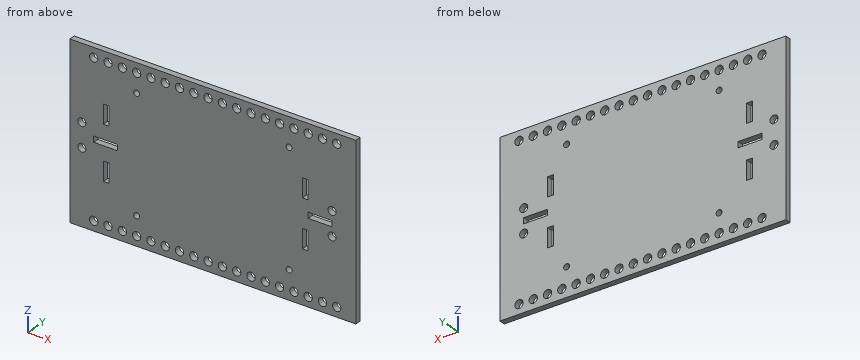
```python
from build123d import *

# Parameters (mm, degrees)
SKETCH1_W           = 152.4
SKETCH1_H           = 91.44
SKETCH1_R           = 2.2225
SKETCH1_R_2         = 2.15265
SKETCH1_R_3         = 1.5875
SKETCH1_W_2         = 12.7
SKETCH1_H_2         = 3.0734
SKETCH1_H_3         = 3.1242
BOSS_EXTRUDE1_DEPTH = 3.175
CUT_EXTRUDE2_REACH  = 90.92
SKETCH2_W           = 3.1242
SKETCH2_H           = 10.1092


with BuildPart() as part:
    # Sketch1 → Boss-Extrude1 (new body)
    with BuildSketch(Plane(origin=(0, 0, 0), x_dir=(1, 0, 0), z_dir=(0, 1, 0))):
        Rectangle(SKETCH1_W, SKETCH1_H)
        with Locations(Location((-63.5, 40.64, 0), (0, 0, 270))):
            Circle(SKETCH1_R, mode=Mode.SUBTRACT)
        with Locations(Location((-63.5, -40.64, 0), (0, 0, 270))):
            Circle(SKETCH1_R, mode=Mode.SUBTRACT)
        with Locations(Location((-69.85, -6.35, 0), (0, 0, 270))):
            Circle(SKETCH1_R_2, mode=Mode.SUBTRACT)
        with Locations(Location((-69.85, 6.35, 0), (0, 0, 270))):
            Circle(SKETCH1_R_2, mode=Mode.SUBTRACT)
        with Locations(Location((63.5, 6.35, 0), (0, 0, 270))):
            Circle(SKETCH1_R_2, mode=Mode.SUBTRACT)
        with Locations(Location((63.5, -6.35, 0), (0, 0, 270))):
            Circle(SKETCH1_R_2, mode=Mode.SUBTRACT)
        with Locations(Location((-55.88, -40.64, 0), (0, 0, 270))):
            Circle(SKETCH1_R, mode=Mode.SUBTRACT)
        with Locations(Location((-55.88, 40.64, 0), (0, 0, 270))):
            Circle(SKETCH1_R, mode=Mode.SUBTRACT)
        with Locations(Location((-48.26, -40.64, 0), (0, 0, 270))):
            Circle(SKETCH1_R, mode=Mode.SUBTRACT)
        with Locations(Location((-48.26, 40.64, 0), (0, 0, 270))):
            Circle(SKETCH1_R, mode=Mode.SUBTRACT)
        with Locations(Location((-40.64, -40.64, 0), (0, 0, 270))):
            Circle(SKETCH1_R, mode=Mode.SUBTRACT)
        with Locations(Location((-40.64, 40.64, 0), (0, 0, 270))):
            Circle(SKETCH1_R, mode=Mode.SUBTRACT)
        with Locations(Location((-33.02, -40.64, 0), (0, 0, 270))):
            Circle(SKETCH1_R, mode=Mode.SUBTRACT)
        with Locations(Location((-33.02, 40.64, 0), (0, 0, 270))):
            Circle(SKETCH1_R, mode=Mode.SUBTRACT)
        with Locations(Location((-25.4, -40.64, 0), (0, 0, 270))):
            Circle(SKETCH1_R, mode=Mode.SUBTRACT)
        with Locations(Location((-25.4, 40.64, 0), (0, 0, 270))):
            Circle(SKETCH1_R, mode=Mode.SUBTRACT)
        with Locations(Location((-17.78, -40.64, 0), (0, 0, 270))):
            Circle(SKETCH1_R, mode=Mode.SUBTRACT)
        with Locations(Location((-17.78, 40.64, 0), (0, 0, 270))):
            Circle(SKETCH1_R, mode=Mode.SUBTRACT)
        with Locations(Location((-10.16, -40.64, 0), (0, 0, 270))):
            Circle(SKETCH1_R, mode=Mode.SUBTRACT)
        with Locations(Location((-10.16, 40.64, 0), (0, 0, 270))):
            Circle(SKETCH1_R, mode=Mode.SUBTRACT)
        with Locations(Location((-2.54, -40.64, 0), (0, 0, 270))):
            Circle(SKETCH1_R, mode=Mode.SUBTRACT)
        with Locations(Location((-2.54, 40.64, 0), (0, 0, 270))):
            Circle(SKETCH1_R, mode=Mode.SUBTRACT)
        with Locations(Location((5.08, -40.64, 0), (0, 0, 270))):
            Circle(SKETCH1_R, mode=Mode.SUBTRACT)
        with Locations(Location((5.08, 40.64, 0), (0, 0, 270))):
            Circle(SKETCH1_R, mode=Mode.SUBTRACT)
        with Locations(Location((12.7, -40.64, 0), (0, 0, 270))):
            Circle(SKETCH1_R, mode=Mode.SUBTRACT)
        with Locations(Location((12.7, 40.64, 0), (0, 0, 270))):
            Circle(SKETCH1_R, mode=Mode.SUBTRACT)
        with Locations(Location((20.32, -40.64, 0), (0, 0, 270))):
            Circle(SKETCH1_R, mode=Mode.SUBTRACT)
        with Locations(Location((20.32, 40.64, 0), (0, 0, 270))):
            Circle(SKETCH1_R, mode=Mode.SUBTRACT)
        with Locations(Location((27.94, -40.64, 0), (0, 0, 270))):
            Circle(SKETCH1_R, mode=Mode.SUBTRACT)
        with Locations(Location((27.94, 40.64, 0), (0, 0, 270))):
            Circle(SKETCH1_R, mode=Mode.SUBTRACT)
        with Locations(Location((35.56, -40.64, 0), (0, 0, 270))):
            Circle(SKETCH1_R, mode=Mode.SUBTRACT)
        with Locations(Location((35.56, 40.64, 0), (0, 0, 270))):
            Circle(SKETCH1_R, mode=Mode.SUBTRACT)
        with Locations(Location((43.18, -40.64, 0), (0, 0, 270))):
            Circle(SKETCH1_R, mode=Mode.SUBTRACT)
        with Locations(Location((43.18, 40.64, 0), (0, 0, 270))):
            Circle(SKETCH1_R, mode=Mode.SUBTRACT)
        with Locations(Location((50.8, -40.64, 0), (0, 0, 270))):
            Circle(SKETCH1_R, mode=Mode.SUBTRACT)
        with Locations(Location((50.8, 40.64, 0), (0, 0, 270))):
            Circle(SKETCH1_R, mode=Mode.SUBTRACT)
        with Locations(Location((58.42, -40.64, 0), (0, 0, 270))):
            Circle(SKETCH1_R, mode=Mode.SUBTRACT)
        with Locations(Location((58.42, 40.64, 0), (0, 0, 270))):
            Circle(SKETCH1_R, mode=Mode.SUBTRACT)
        with Locations(Location((66.04, -40.64, 0), (0, 0, 270))):
            Circle(SKETCH1_R, mode=Mode.SUBTRACT)
        with Locations(Location((66.04, 40.64, 0), (0, 0, 270))):
            Circle(SKETCH1_R, mode=Mode.SUBTRACT)
        with Locations(Location((-40.64, 30.48, 0), (0, 0, 270))):
            Circle(SKETCH1_R_3, mode=Mode.SUBTRACT)
        with Locations(Location((-40.64, -30.48, 0), (0, 0, 270))):
            Circle(SKETCH1_R_3, mode=Mode.SUBTRACT)
        with Locations(Location((40.64, -30.48, 0), (0, 0, 270))):
            Circle(SKETCH1_R_3, mode=Mode.SUBTRACT)
        with Locations(Location((40.64, 30.48, 0), (0, 0, 270))):
            Circle(SKETCH1_R_3, mode=Mode.SUBTRACT)
        with Locations((57.15, 0)):
            Rectangle(SKETCH1_W_2, SKETCH1_H_2, mode=Mode.SUBTRACT)
        with Locations((-57.15, -0.0254)):
            Rectangle(SKETCH1_W_2, SKETCH1_H_3, mode=Mode.SUBTRACT)
    extrude(amount=BOSS_EXTRUDE1_DEPTH)

    # Sketch2 → Cut-Extrude2 (cut, up to next)
    with BuildSketch(Plane(origin=(0, 3.175, 0), x_dir=(1, 0, 0), z_dir=(0, 1, 0)), mode=Mode.PRIVATE) as cut_extrude2_sk1:
        with Locations((-56.8579, 14.2113)):
            Rectangle(SKETCH2_W, SKETCH2_H)
    cut_extrude2_tool1 = extrude(cut_extrude2_sk1.sketch, amount=-CUT_EXTRUDE2_REACH, mode=Mode.PRIVATE) & part.part
    # Sketch2 → Cut-Extrude2 (cut, up to next)
    with BuildSketch(Plane(origin=(0, 3.175, 0), x_dir=(1, 0, 0), z_dir=(0, 1, 0)), mode=Mode.PRIVATE) as cut_extrude2_sk2:
        with Locations((-56.8579, -14.2113)):
            Rectangle(SKETCH2_W, SKETCH2_H)
    cut_extrude2_tool2 = extrude(cut_extrude2_sk2.sketch, amount=-CUT_EXTRUDE2_REACH, mode=Mode.PRIVATE) & part.part
    # Sketch2 → Cut-Extrude2 (cut, up to next)
    with BuildSketch(Plane(origin=(0, 3.175, 0), x_dir=(1, 0, 0), z_dir=(0, 1, 0)), mode=Mode.PRIVATE) as cut_extrude2_sk3:
        with Locations((49.2379, 12.6746)):
            Rectangle(SKETCH2_W, SKETCH2_H)
    cut_extrude2_tool3 = extrude(cut_extrude2_sk3.sketch, amount=-CUT_EXTRUDE2_REACH, mode=Mode.PRIVATE) & part.part
    # Sketch2 → Cut-Extrude2 (cut, up to next)
    with BuildSketch(Plane(origin=(0, 3.175, 0), x_dir=(1, 0, 0), z_dir=(0, 1, 0)), mode=Mode.PRIVATE) as cut_extrude2_sk4:
        with Locations((49.2379, -12.6746)):
            Rectangle(SKETCH2_W, SKETCH2_H)
    cut_extrude2_tool4 = extrude(cut_extrude2_sk4.sketch, amount=-CUT_EXTRUDE2_REACH, mode=Mode.PRIVATE) & part.part
    add(cut_extrude2_tool1.solids().sort_by_distance((-56.8579, 3.175, -14.2113))[0], mode=Mode.SUBTRACT)
    add(cut_extrude2_tool2.solids().sort_by_distance((-56.8579, 3.175, 14.2113))[0], mode=Mode.SUBTRACT)
    add(cut_extrude2_tool3.solids().sort_by_distance((49.2379, 3.175, -12.6746))[0], mode=Mode.SUBTRACT)
    add(cut_extrude2_tool4.solids().sort_by_distance((49.2379, 3.175, 12.6746))[0], mode=Mode.SUBTRACT)


solid = part.part
```
Geometry check sheet. Reference: the model listing, model coordinates, mm. Round coordinates to 2 decimals unless told otherwise and drop trailing zeros. Order: outer loops, then holes, each group sorted by start corner. A loop starts at its lowest first (then second) coordinate and runs counter-clockwise, first axis right, second up. Notation, with made-up numbers: (65, -9.75) - (115, -9.75) arc R27 ccw to (115, 19.25) - close; hole circle Ø1 at (49, 24.5). An arc over 180 degrees is marked (long way). Use a Markdown table: item, result. Add a question column.
1) Section check A-A (x = 12.7). Record the cut outline in (y, z) (1 decimal).
2) Section check B-B (x = 58.42). Record the cut outline in (y, z) (1 decimal).
3) Section check C-C (z = -14.5). Record the cut outline in (x, y) (3 decimals), then the cut area to 3 significant figures.
4) Section check D-D (y = 1.05). Count the separate pieces of the cut face and the enclosed holes in it, then the cut area to 3 significant figures.
5) Gauge pin test, flat ends, axial feed: P1, Ø8, axis at x = -22.5, z = -4.5, coming from the -Y side; P2, Ø3.5, axis at x = -17.78, z = -40.64, coming from the -Y side. Record the tip position at first contact, or that the pin passes through.
6) Thickness scan on line 1 along Z through (x, y) = (66, 1); line 2 along Z through (x, y) = (67.5, 1.5); line 3 along X through (y, z) = (2.6, 30). Record the ranges inside material, lowest first.
Established:
| question | item | result |
|---|---|---|
| 1 | outline | (0, -45.7) - (3.2, -45.7) - (3.2, -42.9) - (0, -42.9) - close; (0, -38.4) - (3.2, -38.4) - (3.2, 38.4) - (0, 38.4) - close; (0, 42.9) - (3.2, 42.9) - (3.2, 45.7) - (0, 45.7) - close |
| 2 | outline | (0, -45.7) - (3.2, -45.7) - (3.2, -42.9) - (0, -42.9) - close; (0, -38.4) - (3.2, -38.4) - (3.2, -1.5) - (0, -1.5) - close; (0, 1.5) - (3.2, 1.5) - (3.2, 38.4) - (0, 38.4) - close; (0, 42.9) - (3.2, 42.9) - (3.2, 45.7) - (0, 45.7) - close |
| 3 | outline | (-76.2, 0) - (-58.42, 0) - (-58.42, 3.175) - (-76.2, 3.175) - close; (-55.296, 0) - (47.676, 0) - (47.676, 3.175) - (-55.296, 3.175) - close; (50.8, 0) - (76.2, 0) - (76.2, 3.175) - (50.8, 3.175) - close |
| 3 | area | 464 mm2 |
| 4 | separate pieces | 1 |
| 4 | enclosed holes | 50 |
| 4 | area | 13,100 mm2 |
| 5 | P1 | y = 0 |
| 5 | P2 | through |
| 6 | line 1 | -45.72 to -42.86, -38.42 to 38.42, 42.86 to 45.72 |
| 6 | line 2 | -45.72 to -42.32, -38.96 to 38.96, 42.32 to 45.72 |
| 6 | line 3 | -76.2 to -42.15, -39.13 to 39.13, 42.15 to 76.2 |
